```python
from build123d import *

# Parameters (mm, degrees)
SKETCH1_R           = 20
SKETCH1_R_2         = 15
BOSS_EXTRUDE1_DEPTH = 15
SKETCH2_R           = 30
SKETCH2_R_2         = 20
BOSS_EXTRUDE2_DEPTH = 7.5
SKETCH3_W           = 6
SKETCH3_H           = 34.327772866
CUT_EXTRUDE1_DEPTH  = 16


with BuildPart() as part:
    # Sketch1 → Boss-Extrude1 (new body)
    with BuildSketch(Plane.XY):
        Circle(SKETCH1_R)
        Circle(SKETCH1_R_2, mode=Mode.SUBTRACT)
    extrude(amount=BOSS_EXTRUDE1_DEPTH)

    # Sketch2 → Boss-Extrude2 (add)
    with BuildSketch(Plane(origin=(0, 0, 0), x_dir=(-1, 0, 0), z_dir=(0, 0, -1))):
        Circle(SKETCH2_R)
        Circle(SKETCH2_R_2, mode=Mode.SUBTRACT)
    extrude(amount=-BOSS_EXTRUDE2_DEPTH)

    # Sketch3 → Cut-Extrude1 (cut, through all)
    with BuildSketch(Plane.XY):
        with Locations((0, 17.163886433)):
            Rectangle(SKETCH3_W, SKETCH3_H)
    extrude(amount=CUT_EXTRUDE1_DEPTH, mode=Mode.SUBTRACT)


solid = part.part
```
Source: CAD feature listing. Evaluate the final solid. Frame: model axes, mm. A direction names the side the tool comes from. Give positions to 0.01 mm unless a question says otherwise; leave off trailing zeros. Write each loop counter-clockwise with the first axis right and the second up, starting at its lowest first coordinate (ties: lowest second). Pieces come first, ordered by that corner, then holes.
1. Section query A-A (y = 0). Return the cut outline in (x, z), then the cut area to 3 significant figures.
2. Section query B-B (x = 12). Return the cut outline in (y, z), then the cut area to 3 significant figures.
3. Material intervals for line 1 along X through (y, z) = (0, 13.5); line 2 along X through (y, z) = (0, 5); line 3 along Y through (x, z) = (0, 7), sorted ascending.
4. First-contact query: pin 1 (7.5 mm diameter, centred on y = 21, z = 10, fed in from -X); pin 2 (4.5 mm diameter, centred on y = 19, z = 6, fed in from +X); pin 3 (1.5 mm diameter, centred on x = 23.5, y = -11.5, fed in from +Z). Flat tips, straight axial feed; report the tip coordinate or a pass-through.
5. Pull-direction query (X, two-part tool) for faces 1 (the face through (14, -6, 0)), 2 (the face through (1.277, -29.973, 3.698)), 3 (the face through (-3, 20, 6)); classes: +X half, -X half, draft (parallel to the pull), parting line (faces both ways), or undercut.
6. Section query C-C (x = 0). Return the cut outline in (y, z).
7. Section query D-D (y = -24). Return the cut outline in (x, z).
8. Access query for faces 4 (the face through (-0.837, -19.982, 11.198)), 5 (the face through (-3, -15, 15)), 6 (the face through (3, 20, 6)). Directions: +Z, -Z, +X, -X, +Y, -Y. A direction counts if a zero-diameter tool reaches every point of the face in a straight line with its end or side. Return the directions, or none.
Output values:
1. outline: (-30, 0) - (-15, 0) - (-15, 15) - (-20, 15) - (-20, 7.5) - (-30, 7.5) - close; (15, 0) - (30, 0) - (30, 7.5) - (20, 7.5) - (20, 15) - (15, 15) - close
1. area: 300 mm2
2. outline: (-27.5, 0) - (-9, 0) - (-9, 15) - (-16, 15) - (-16, 7.5) - (-27.5, 7.5) - close; (9, 0) - (27.5, 0) - (27.5, 7.5) - (16, 7.5) - (16, 15) - (9, 15) - close
2. area: 382 mm2
3. line 1: x = -20 to -15, 15 to 20
3. line 2: x = -30 to -15, 15 to 30
3. line 3: y = -30 to -15
4. pin 1: stops at x = -23.84
4. pin 2: stops at x = 24.89
4. pin 3: stops at z = 7.5
5. face 1: draft
5. face 2: parting line
5. face 3: undercut
6. outline: (-30, 0) - (-15, 0) - (-15, 15) - (-20, 15) - (-20, 7.5) - (-30, 7.5) - close
7. outline: (-18, 0) - (18, 0) - (18, 7.5) - (-18, 7.5) - close
8. face 4: +Z
8. face 5: +Z, +X, -X, +Y, -Y
8. face 6: +Z, -Z, +Y
